from build123d import *

# Parameters (mm, degrees)
FILLET1_R   = 0.2
HEX_START   = -1.9
HEX_2_DEPTH = 1.9


with BuildPart() as part:
    # BodySke → BaseBody (revolve)
    with BuildSketch(Plane.XY, mode=Mode.PRIVATE) as basebody_sk:
        Polygon((0, 0), (0, 4.875), (0.725, 4.875), (3.1, 2.5), (39.555, 2.5), (40, 2.055), (40, 0), align=None)
    revolve(basebody_sk.sketch.rotate(Axis((0, 0, 0), (1, 0, 0)), 90), axis=Axis((0, 0, 0), (1, 0, 0)))

    # Fillet1
    fillet1_edges = [part.edges().sort_by_distance(p)[0] for p in [
        (3.1, 0, -2.5),
    ]]
    fillet(fillet1_edges, radius=FILLET1_R)

    # Hex 2: read off the stored shape, not the designer's step
    # Hex 2 outline → Hex 2 (cut)
    with BuildSketch(Plane.ZY.offset(HEX_START)):
        Polygon((-1.5, -0.866025404), (0, -1.732050808), (1.5, -0.866025404), (1.5, 0.866025404), (0, 1.732050808), (-1.5, 0.866025404), align=None)
    extrude(amount=HEX_2_DEPTH, mode=Mode.SUBTRACT)

    # Hex 2 2 outline → Hex 2 2 (revolve, cut)
    with BuildSketch(Plane.YX):
        Polygon((1.5, 1.9), (0, 2.766025404), (0, 1.9), align=None)
    revolve(axis=Axis((0, 0, 0), (1, 0, 0)), mode=Mode.SUBTRACT)


solid = part.part
Geometry check sheet. Reference: the model listing, model coordinates, mm. A direction names the side the tool comes from. Round coordinates to 2 decimals unless told otherwise and drop trailing zeros. Write each loop counter-clockwise with the first axis right and the second up, starting at its lowest first coordinate (ties: lowest second). Pieces come first, ordered by that corner, then holes. Notation, with made-up numbers: (-26.5, -12.75) -> (16.5, -12.75) arc R20 cw to (16.5, -8.75) -> close; hole circle Ø3 at (1.5, 32). An arc over 180 degrees is marked (long way). One line per item, written item: value. Start each with the question number.
(1) Cross-section at A-A, the plane x = 25. Record the cut outline in (y, z), and give its area (3 significant figures).
(2) Scan lines: line 1 (X direction, y = -0.75, z = 2.5); line 2 (Y direction, x = 30, z = -2); line 3 (X direction, y = 0.5, z = -2.25). Record each from-to range of solid material in increasing order. Write a range as [from, to].
(3) Draft check along Z on faces 4 (the conical face through (2.93, -0.8, 2.55)), 5 (the conical face through (2.63, -0.05, -0.23)), 6 (the flat face through (0, 0, -2)). Enter one of: +Z half, -Z half, draft (parallel to the pull), parting line (faces both ways), or undercut.
(4) Go/stop test with flat-tipped pins: pin 1 Ø1.5 at (x, y) = (7.5, 0) entering from +Z; pin 2 Ø1.5 at (x, z) = (30.5, -1.5) entering from -Y; pin 3 Ø0.6 at (y, z) = (-0.5, 1) entering from -X. Record where each tip stops, or that it passes through.
(5) Access from +Z, -Z, +X, -X, +Y, -Y to the whole of each face (thin tool, end or side, straight path). Record for faces 1 (the cylindrical face through (21.624, -0.751, 2.385)), 2 (the cylindrical face through (0.368, -4.834, -0.635)), 3 (the flat face through (0.963, 1.305, -0.74)).
Answer:
1. outline: circle Ø5 at (0, 0)
1. area: 19.6 mm²
2. line 1: [0, 2.99]
2. line 2: [-1.5, 1.5]
2. line 3: [0, 39.75]
3. face 4: parting line
3. face 5: undercut
3. face 6: draft
4. pin 1: z = 2.5
4. pin 2: y = -2.38
4. pin 3: x = 1.95
5. face 1: +X
5. face 2: +X, -X
5. face 3: -X
